Part print with two shaded views. Sizes in mm from the minimum x, y, z corner. A direction names the side the tool comes from. Coordinates: 2 decimals unless noted, no trailing zeros. Write each loop counter-clockwise with the first axis right and the second up, starting at its lowest first coordinate (ties: lowest second). Pieces come first, ordered by that corner, then holes. Notation, with made-up numbers: (-32, 50) - (22, 50) arc R7 cw to (22, 58) - close; hole circle Ø11 at (-27.5, 38.25). An arc over 180 degrees is marked (long way). One line per question, with ' | ' between items. Start each with the question number.
1. Band-saw the part on C-C, the plane x = 55. Write the cut outline in (y, z), then the cut area to 3 significant figures.
2. Two-plate mould, pull along Y, no slides. Class the marked faces 1, 2 and 3: +Y half, -Y half, draft (parallel to the pull), parting line (faces both ways), or undercut.
3. Flat gauge pins, fed straight in: P1, Ø15, axis at x = 19.05, y = 19.05, coming from the +Z side; P2, Ø13.5, axis at x = 80, z = 13.5, coming from the -Y side; P3, Ø3, axis at y = 31.5, z = 36.5, coming from the -X side; P4, Ø12, axis at y = 7.5, z = 39.5, coming from the +X side. Where does each tip first touch, or does it go through?
4. Probe line 1 (X direction, y = 19.05, z = 18.5) (3 decimals); line 2 (Y direction, x = 19, z = 28); line 3 (Z direction, x = 74, y = 33). List the from-to ranges inside material, lowest first.
5. Which spindle directions (+Z, -Z, +X, -X, +Y, -Y) get a long thin tool onto all of the face, cutting with end or side? Do the marked faces 4, 5 and 6. Say none if no direction does.
6. Band-saw the part on A-A, the plane x = 86.5. Write the cut outline in (y, z), then the cut area to 3 significant figures.
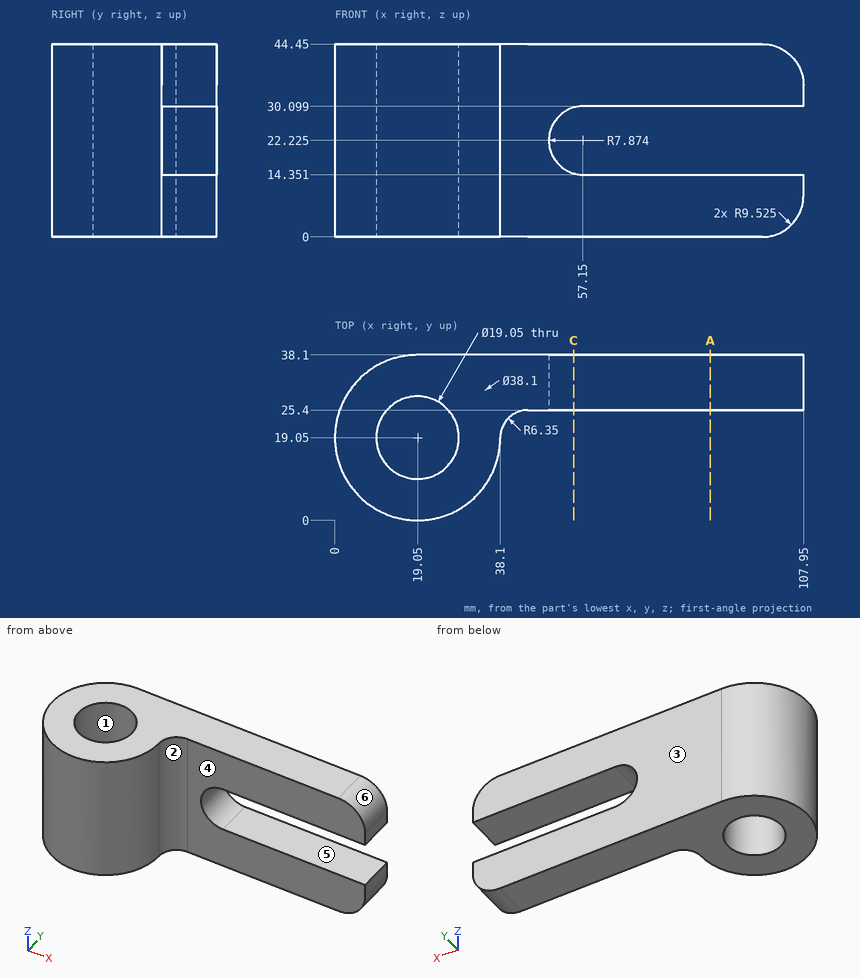
Filled in:
1) outline: (25.4, 0) - (38.1, 0) - (38.1, 14.65) - (25.4, 14.65) - close; (25.4, 29.8) - (38.1, 29.8) - (38.1, 44.45) - (25.4, 44.45) - close | area: 372 mm²
2) face 1: undercut | face 2: -Y half | face 3: +Y half
3) P1: passes through | P2: stops at y = 25.4 | P3: stops at x = 3.46 | P4: stops at x = 37.27
4) line 1: x = 0 to 9.525, 28.575 to 38.1 | line 2: y = 0 to 9.53, 28.57 to 38.1 | line 3: z = 0 to 14.35, 30.1 to 44.45
5) face 4: +Z, -Z, +X, -Y | face 5: +X, +Y, -Y | face 6: +Z, +X, +Y, -Y
6) outline: (25.4, 0) - (38.1, 0) - (38.1, 14.35) - (25.4, 14.35) - close; (25.4, 30.1) - (38.1, 30.1) - (38.1, 44.45) - (25.4, 44.45) - close | area: 365 mm²
